Print and shaded views of the part. All mm, measured from the part's lowest x, y and z. Coordinates: 2 decimals unless noted, no trailing zeros. Order: outer loops, then holes, each group sorted by start corner. A loop starts at its lowest first (then second) coordinate and runs counter-clockwise, first axis right, second up. Notation, with made-up numbers: (84.5, 88) -> (143.5, 88) arc R11 cw to (143.5, 103) -> close; hole circle Ø10 at (84, 62). An arc over 180 degrees is marked (long way). Return JSON: item names as keys, results as strings. Group by question number.
1) Cut at A-A (y = 30.5). Write the cut outline in (x, z).
2) Cut at B-B (x = 26.5). Write the cut outline in (y, z).
3) Probe line 1 (Y direction, x = 62.5, z = 2.1); line 2 (X direction, y = 51.5, z = 2.35). List the from-to ranges inside material, lowest first.
4) Flat gauge pins, fed straight in: pin 1 (1.6 mm diameter, centred on x = 54, z = 1, fed in from -Y); pin 2 (1 mm diameter, centred on y = 80.5, z = 2.5, fed in from -X); pin 3 (1 mm diameter, centred on x = 1.5, z = 2, fed in from -Y); pin 4 (1 mm diameter, centred on y = 72.5, z = 2, fed in from +X). Where does each tip first touch, or does it go through?
5) Cut at C-C (z = 0.55). State how many separate pieces and enclosed holes the cut face has, and give its area (3 significant figures).
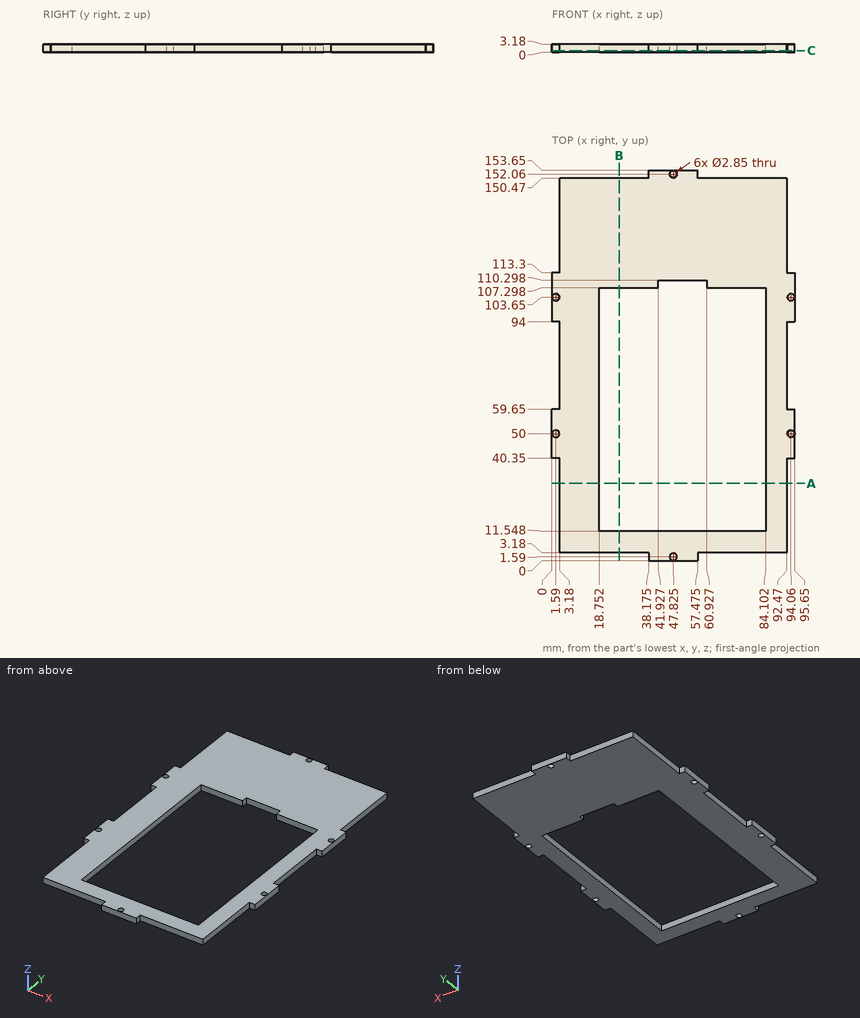
Answers below:
{
 "1": {"outline": "(3.18, 0) -> (18.75, 0) -> (18.75, 3.18) -> (3.18, 3.18) -> close; (84.1, 0) -> (92.47, 0) -> (92.47, 3.18) -> (84.1, 3.18) -> close"},
 "2": {"outline": "(3.18, 0) -> (11.55, 0) -> (11.55, 3.18) -> (3.18, 3.18) -> close; (107.3, 0) -> (150.47, 0) -> (150.47, 3.18) -> (107.3, 3.18) -> close"},
 "3": {"line 1": "y = 3.18 to 11.55, 107.3 to 150.47", "line 2": "x = 0 to 18.75, 84.1 to 95.65"},
 "4": {"pin 1": "stops at y = 0", "pin 2": "stops at x = 3.18", "pin 3": "stops at y = 40.35", "pin 4": "stops at x = 92.47"},
 "5": {"separate pieces": "1", "enclosed holes": "7", "area": "7,170 mm^2"}
}
